Could you check a few things on this model? Use its own coordinates, in mm. A direction names the side the tool comes from. Round coordinates to 2 decimals unless told otherwise and drop trailing zeros. Write each loop counter-clockwise with the first axis right and the second up, starting at its lowest first coordinate (ties: lowest second). Pieces come first, ordered by that corner, then holes. Notation, with made-up numbers: (86.5, 16.25) -> (104.5, 16.25) arc R17 cw to (104.5, 49.25) -> close; hole circle Ø9 at (-1, 27). An arc over 180 degrees is marked (long way). Answer as CSV lines item,"result". Start each with the question number.
Q1. For faces 3 (the flat face through (42, 0, 57)), 4 (the flat face through (50, -8, 51)), 5 (the cylindrical face through (-7.5, 0.1, 46.7)), which set-ups out of +Z, -Z, +X, -X, +Y, -Y let a thin tool reach every point of the face, with its end or its side?
Q2. If I drill on line 1 (X direction, y = -25, z = 56.75); line 2 (Y direction, x = -18, z = 53.5); line 3 (X direction, y = -17, z = 45.5), over which ranges is the centre line in solid material (lowest first)? Write a range as [from, to].
Q3. Imagine slicing it at A-A on z = 53.25. Give the number of separate pieces and of enclosed holes in the cut face, and give its area (4 significant figures).
Q4. Imagine slicing it at D-D on y = -15.5. Please give me the cut outline in (x, z).
Q5. If we mould it in two halves opening along Y, with no side actions, what happens to faces 1 (the flat face through (-42, 0, 52)), 2 (the flat face through (-10, -22, 62.7))? For each: pulls with the +Y half, pulls with the -Y half, needs draft (parallel to the pull), parting line crosses it, or undercut.
Q6. Will these pins go through, and if not, where does the flat tip stop? pin 1 Ø2 at (x, y) = (-18.5, -25.5) entering from +Z; pin 2 Ø3 at (x, y) = (-18, 16.5) entering from +Z; pin 3 Ø1 at (y, z) = (8.5, 59) entering from +X.
Q7. Imagine slicing it at B-B on x = 50. Please give me the cut outline in (y, z).
Q8. Imagine slicing it at C-C on y = 0. Please give me the cut outline in (x, z).
from build123d import *

# Parameters (mm, degrees)
PAD_DEPTH       = 29
POCKET_DEPTH    = 21
SKETCH003_R     = 2
SKETCH003_R_2   = 4
PAD002_DEPTH    = 4.5
SKETCH007_R     = 2
POCKET002_DEPTH = 16.5
SKETCH008_W     = 36
SKETCH008_H     = 55.8
POCKET003_DEPTH = 12.6
POCKET004_DEPTH = 1
PAD005_DEPTH    = 11.2
SKETCH011_W     = 8
SKETCH011_H     = 16
POCKET005_DEPTH = 16
PAD013_DEPTH    = 2.7


with BuildPart() as part:
    # Sketch → Pad (new body, symmetric)
    with BuildSketch(Plane.XZ):
        Polygon((-32, 0), (44, 0), (44, 16.5), (-44, 16.5), (-44, -5.5), (-32, -5.5), align=None)
    extrude(amount=PAD_DEPTH, both=True)

    # Sketch002 → Pocket (cut, symmetric)
    with BuildSketch(Plane.XZ):
        Polygon((-42, 16.5), (-42, -4.5), (-34, -4.5), (-34, 1), (42, 1), (42, 16.5), align=None)
    extrude(amount=POCKET_DEPTH, both=True, mode=Mode.SUBTRACT)

    # Sketch003 (on DatumPlane) → Pad002 (join)
    with BuildSketch(Plane.XY.offset(1)):
        with Locations((-17, 15.5)):
            Circle(SKETCH003_R)
        with Locations((-6, -15.5)):
            Circle(SKETCH003_R_2)
        with Locations((-6, -15.5)):
            Circle(SKETCH003_R, mode=Mode.SUBTRACT)
        with Locations((-28, -15.5)):
            Circle(SKETCH003_R_2)
        with Locations((-28, -15.5)):
            Circle(SKETCH003_R, mode=Mode.SUBTRACT)
    extrude(amount=PAD002_DEPTH)

    # Sketch007 (on DatumPlane) → Pocket002 (cut)
    with BuildSketch(Plane.XY.offset(1)):
        with Locations((-40, 25)):
            Circle(SKETCH007_R)
        with Locations((-18, 25)):
            Circle(SKETCH007_R)
        with Locations((40, 25)):
            Circle(SKETCH007_R)
        with Locations((40, -25)):
            Circle(SKETCH007_R)
        with Locations((-40, -25)):
            Circle(SKETCH007_R)
        with Locations((-18, -25)):
            Circle(SKETCH007_R)
    extrude(amount=POCKET002_DEPTH, mode=Mode.SUBTRACT)

    # Sketch008 (on DatumPlane) → Pocket003 (cut)
    with BuildSketch(Plane.XY.offset(16.5)):
        with Locations((18, 0)):
            Rectangle(SKETCH008_W, SKETCH008_H)
    extrude(amount=-POCKET003_DEPTH, mode=Mode.SUBTRACT)

    # Sketch009 (on DatumPlane) → Pocket004 (cut)
    with BuildSketch(Plane.XY.offset(1)):
        with BuildLine():
            ThreePointArc((-2.5, 5), (-7.5, 0), (-2.5, -5))
            Line((-2.5, -5), (12.5, -5))
            ThreePointArc((12.5, -5), (17.5, 0), (12.5, 5))
            Line((12.5, 5), (-2.5, 5))
        make_face()
    extrude(amount=-POCKET004_DEPTH, mode=Mode.SUBTRACT)

    # Sketch010 → Pad005 (join)
    with BuildSketch(Plane.XY):
        with BuildLine():
            Line((45.5, 9.6), (58.5, 9.6))
            ThreePointArc((60, 8.1), (59.56066, 9.16066), (58.5, 9.6))
            Line((60, 8.1), (60, -8.1))
            ThreePointArc((58.5, -9.6), (59.56066, -9.16066), (60, -8.1))
            Line((58.5, -9.6), (45.5, -9.6))
            ThreePointArc((45.5, -9.6), (44.43934, -10.03934), (44, -11.1))
            Line((44, 11.1), (44, -11.1))
            ThreePointArc((44, 11.1), (44.43934, 10.03934), (45.5, 9.6))
        make_face()
    extrude(amount=PAD005_DEPTH)

    # Sketch011 (on DatumPlane) → Pocket005 (cut)
    with BuildSketch(Plane(origin=(42, 0, 0), x_dir=(0, 0, -1), z_dir=(1, 0, 0))):
        with Locations((-5, 0)):
            Rectangle(SKETCH011_W, SKETCH011_H)
    extrude(amount=POCKET005_DEPTH, mode=Mode.SUBTRACT)

    # Sketch019 → Pad013 (join)
    with BuildSketch(Plane.XY):
        Polygon((-32, 27.8), (44, 27.8), (44, 29), (-32.4, 29), (-32.4, -29), (44, -29), (44, -27.8), (-32, -27.8), align=None)
    extrude(amount=-PAD013_DEPTH)


with BuildPart() as part_1:
    # Body placement: moved
    add(part.part.moved(Location((0, 0, 46.2))))


solid = part_1.part
Checks:
1,face 3,"+Z"
1,face 4,"none"
1,face 5,"+Z, -Z"
2,line 1,"[-44, -42], [-38, -20], [-16, 0], [36, 38], [42, 44]"
2,line 2,"[-29, -27], [-23, -21], [21, 23], [27, 29]"
2,line 3,"[-44, -42], [-34, -32]"
3,separate pieces,"1"
3,enclosed holes,"7"
3,area,"1,055 mm^2"
4,outline,"(-44, 40.7) -> (-32, 40.7) -> (-32, 46.2) -> (44, 46.2) -> (44, 62.7) -> (42, 62.7) -> (42, 47.2) -> (-2, 47.2) -> (-2, 51.7) -> (-4, 51.7) -> (-4, 47.2) -> (-8, 47.2) -> (-8, 51.7) -> (-10, 51.7) -> (-10, 47.2) -> (-24, 47.2) -> (-24, 51.7) -> (-26, 51.7) -> (-26, 47.2) -> (-30, 47.2) -> (-30, 51.7) -> (-32, 51.7) -> (-32, 47.2) -> (-34, 47.2) -> (-34, 41.7) -> (-42, 41.7) -> (-42, 62.7) -> (-44, 62.7) -> close"
5,face 1,"undercut"
5,face 2,"needs draft"
6,pin 1,"z = 47.2"
6,pin 2,"z = 51.7"
6,pin 3,"x = 44"
7,outline,"(-9.6, 46.2) -> (9.6, 46.2) -> (9.6, 57.4) -> (-9.6, 57.4) -> close; hole (-8, 47.2) -> (8, 47.2) -> (8, 55.2) -> (-8, 55.2) -> close"
8,outline,"(-44, 40.7) -> (-32, 40.7) -> (-32, 46.2) -> (-7.5, 46.2) -> (-7.5, 47.2) -> (-34, 47.2) -> (-34, 41.7) -> (-42, 41.7) -> (-42, 62.7) -> (-44, 62.7) -> close; (17.5, 46.2) -> (60, 46.2) -> (60, 57.4) -> (44, 57.4) -> (44, 62.7) -> (42, 62.7) -> (42, 55.2) -> (58, 55.2) -> (58, 47.2) -> (17.5, 47.2) -> close"
